```python
from build123d import *

# Parameters (mm, degrees)
BOSS_EXTRUDE2_DEPTH = 6.35
SKETCH6_W           = 2.54
SKETCH6_H           = 7.62
SKETCH6_W_2         = 1.905
CUT_EXTRUDE3_DEPTH  = 6.35
SKETCH7_R           = 10.795
SKETCH7_R_2         = 1.5
CUT_EXTRUDE4_DEPTH  = 6.35
SKETCH10_R          = 7.62
CUT_EXTRUDE6_DEPTH  = 6.35
SKETCH11_W          = 3.81
SKETCH11_H          = 7.62
CUT_EXTRUDE7_DEPTH  = 1.27
SKETCH8_R           = 2
SKETCH8_R_2         = 1.989430384
CUT_EXTRUDE8_DEPTH  = 6.35
SKETCH12_R          = 2
CUT_EXTRUDE9_DEPTH  = 6.35


with BuildPart() as part:
    # Sketch3 → Boss-Extrude2 (new body)
    with BuildSketch(Plane(origin=(0, 0, 0), x_dir=(1, 0, 0), z_dir=(0, 1, 0))):
        with BuildLine():
            Line((-27.819999986, -50.8), (-16.461471842, -50.8))
            Line((-16.461471842, -50.8), (4.000849576, -50.8))
            Line((4.000849576, -50.8), (23.297417358, -50.8))
            Line((23.297417358, -50.8), (27.819999986, -50.8))
            ThreePointArc((27.819999986, -50.8), (29.61605121, -50.056051224), (30.359999986, -48.26))
            Line((30.359999986, -48.26), (30.359999986, -11.643560444))
            ThreePointArc((30.359999986, -11.643560444), (30.670062071, -10.427428504), (31.524548724, -9.508207119))
            ThreePointArc((31.524548724, -9.508207119), (35.329369206, -5.415138673), (36.709999986, 0))
            Line((36.709999986, 0), (36.709999986, 16.964999979))
            ThreePointArc((36.709999986, 16.964999979), (31.054999993, 22.619999972), (25.4, 16.964999979))
            Line((25.4, 16.964999979), (25.4, 11.309999986))
            ThreePointArc((25.4, 11.309999986), (19.514906714, 9.658249153), (15.348771474, 5.185451262))
            ThreePointArc((15.348771474, 5.185451262), (14.413140747, 4.180950232), (13.091466391, 3.81))
            Line((13.091466391, 3.81), (-13.091466391, 3.81))
            ThreePointArc((-13.091466391, 3.81), (-14.413140747, 4.180950232), (-15.348771474, 5.185451262))
            ThreePointArc((-15.348771474, 5.185451262), (-19.514906714, 9.658249153), (-25.4, 11.309999986))
            Line((-25.4, 11.309999986), (-25.4, 16.964999979))
            ThreePointArc((-25.4, 16.964999979), (-31.054999993, 22.619999972), (-36.709999986, 16.964999979))
            Line((-36.709999986, 16.964999979), (-36.709999986, 0))
            ThreePointArc((-36.709999986, 0), (-35.329369206, -5.415138673), (-31.524548724, -9.508207119))
            ThreePointArc((-31.524548724, -9.508207119), (-30.670062071, -10.427428504), (-30.359999986, -11.643560444))
            Line((-30.359999986, -11.643560444), (-30.359999986, -48.26))
            ThreePointArc((-30.359999986, -48.26), (-29.61605121, -50.056051224), (-27.819999986, -50.8))
        make_face()
    extrude(amount=BOSS_EXTRUDE2_DEPTH)

    # Sketch6 → Cut-Extrude3 (cut)
    with BuildSketch(Plane(origin=(0, 6.35, 0), x_dir=(1, 0, 0), z_dir=(0, 1, 0))):
        with Locations((-5.08, -3.81)):
            Rectangle(SKETCH6_W, SKETCH6_H)
        with Locations((4.7625, -3.81)):
            Rectangle(SKETCH6_W_2, SKETCH6_H)
        with Locations((10.4775, -3.81)):
            Rectangle(SKETCH6_W_2, SKETCH6_H)
    extrude(amount=-CUT_EXTRUDE3_DEPTH, mode=Mode.SUBTRACT)

    # Sketch7 → Cut-Extrude4 (cut)
    with BuildSketch(Plane(origin=(0, 6.35, 0), x_dir=(1, 0, 0), z_dir=(0, 1, 0))):
        with Locations((-12.7, -36.83)):
            Circle(SKETCH7_R)
        with Locations((12.7, -36.83)):
            Circle(SKETCH7_R_2)
    extrude(amount=-CUT_EXTRUDE4_DEPTH, mode=Mode.SUBTRACT)

    # Sketch10 → Cut-Extrude6 (cut)
    with BuildSketch(Plane(origin=(0, 6.35, 0), x_dir=(1, 0, 0), z_dir=(0, 1, 0))):
        with Locations((-25.4, 0)):
            Circle(SKETCH10_R)
        with Locations((25.4, 0)):
            Circle(SKETCH10_R)
    extrude(amount=-CUT_EXTRUDE6_DEPTH, mode=Mode.SUBTRACT)

    # Sketch11 → Cut-Extrude7 (cut)
    with BuildSketch(Plane(origin=(0, 6.35, 0), x_dir=(1, 0, 0), z_dir=(0, 1, 0))):
        with Locations((7.62, -3.81)):
            Rectangle(SKETCH11_W, SKETCH11_H)
    extrude(amount=-CUT_EXTRUDE7_DEPTH, mode=Mode.SUBTRACT)

    # Sketch8 → Cut-Extrude8 (cut)
    with BuildSketch(Plane(origin=(0, 6.35, 0), x_dir=(1, 0, 0), z_dir=(0, 1, 0))):
        with Locations((-31.75, 15.24)):
            Circle(SKETCH8_R)
        with Locations((-25.4, -15.24)):
            Circle(SKETCH8_R)
        with Locations((25.4, -15.24)):
            Circle(SKETCH8_R_2)
        with Locations((31.75, 15.24)):
            Circle(SKETCH8_R)
    extrude(amount=-CUT_EXTRUDE8_DEPTH, mode=Mode.SUBTRACT)

    # Sketch12 → Cut-Extrude9 (cut)
    with BuildSketch(Plane(origin=(0, 6.35, 0), x_dir=(1, 0, 0), z_dir=(0, 1, 0))):
        with Locations((15.301414721, -14.889872981)):
            Circle(SKETCH12_R)
        with Locations((20.301414721, -23.550127019)):
            Circle(SKETCH12_R)
        with Locations((-22.133830064, -48.050127019)):
            Circle(SKETCH12_R)
        with Locations((-27.133830064, -39.389872981)):
            Circle(SKETCH12_R)
    extrude(amount=-CUT_EXTRUDE9_DEPTH, mode=Mode.SUBTRACT)


solid = part.part
```
CAD build for the part. Positions are in the model's coordinates, mm. A direction names the side the tool comes from. Coordinates: 2 decimals unless noted, no trailing zeros. Write each loop counter-clockwise with the first axis right and the second up, starting at its lowest first coordinate (ties: lowest second). Pieces come first, ordered by that corner, then holes.
(1) Cut at D-D, the plane x = 24.5. List the corners of the cut face in (y, z).
(2) 3-axis set-ups, long thin cutter, end or side, ignore diameter. For faces 1 (the face through (-1, 6.35, 14)), 2 (the face through (7.6, 5.3, 7.62)), 3 (the face through (25.4, 3, -14)), 4 (the face through (5.715, 3, 4)), 5 (the face through (30.36, 3, 30)): which of +Z, -Z, +X, -X, +Y, -Y reach the whole face in a straight line?
(3) Flat gauge pins, fed straight in: pin 1 (2 mm diameter, centred on y = 2.5, z = 7, fed in from -X); pin 2 (3 mm diameter, centred on y = 2, z = 4, fed in from -X); pin 3 (1 mm diameter, centred on x = -1.5, y = 5.5, fed in from -Z). Where does each tip first touch, or does it go through?
(4) Cut at C-C, the plane x = -22.5. List the corners of the cut face in (y, z), and give its area (3 significant figures).
(5) Cut at B-B, the plane z = 5. List the corners of the cut face in (x, y) (3 decimals).
(6) Cut at A-A, the plane z = -15.24. List the corners of the cut face in (x, y).
(7) Two-plate mould, pull along X, no slides. Class faces 6 (the face through (19.589, 3.131, -9.703)), 7 (the face through (0, 3, 50.8)), 8 (the face through (-35.367, 3.131, 5.346)), 9 (the face through (35.291, 3.131, 5.484)): +X half, -X half, draft (parallel to the pull), parting line (faces both ways), or undercut.
(8) Drill centre lines: probe 1 along X at (y, z) = (3.25, -15.24); probe 2 along X at (y, z) = (4.25, 36.83) (3 decimals); probe 3 along Z at (x, y) = (10, 5.25). Where is each one in solid material? Low to high.
Geometry says:
1. outline: (0, -11.27) - (6.35, -11.27) - (6.35, -7.57) - (0, -7.57) - close; (0, 7.57) - (6.35, 7.57) - (6.35, 13.47) - (0, 13.47) - close; (0, 17.01) - (6.35, 17.01) - (6.35, 50.8) - (0, 50.8) - close
2. face 1: +Z, -Z, +X, -X, +Y
2. face 2: +Y
2. face 3: -Z, +Y, -Y
2. face 4: +Y, -Y
2. face 5: +Z, +X, +Y, -Y
3. pin 1: stops at x = -34.99
3. pin 2: stops at x = -36.43
3. pin 3: stops at z = -3.81
4. outline: (0, -10.93) - (6.35, -10.93) - (6.35, -7.05) - (0, -7.05) - close; (0, 7.05) - (6.35, 7.05) - (6.35, 32.3) - (0, 32.3) - close; (0, 41.36) - (6.35, 41.36) - (6.35, 46.08) - (0, 46.08) - close; (0, 50.02) - (6.35, 50.02) - (6.35, 50.8) - (0, 50.8) - close
4. area: 220 mm2
5. outline: (-35.545, 0) - (-31.15, 0) - (-31.15, 6.35) - (-35.545, 6.35) - close; (-19.65, 0) - (-6.35, 0) - (-6.35, 6.35) - (-19.65, 6.35) - close; (-3.81, 0) - (3.81, 0) - (3.81, 6.35) - (-3.81, 6.35) - close; (5.715, 0) - (9.525, 0) - (9.525, 5.08) - (5.715, 5.08) - close; (11.43, 0) - (19.65, 0) - (19.65, 6.35) - (11.43, 6.35) - close; (31.15, 0) - (35.545, 0) - (35.545, 6.35) - (31.15, 6.35) - close
6. outline: (-36.71, 0) - (-33.75, 0) - (-33.75, 6.35) - (-36.71, 6.35) - close; (-29.75, 0) - (-25.4, 0) - (-25.4, 6.35) - (-29.75, 6.35) - close; (25.4, 0) - (29.75, 0) - (29.75, 6.35) - (25.4, 6.35) - close; (33.75, 0) - (36.71, 0) - (36.71, 6.35) - (33.75, 6.35) - close
7. face 6: undercut
7. face 7: draft
7. face 8: -X half
7. face 9: +X half
8. probe 1: x = -36.71 to -33.75, -29.75 to -25.4, 25.4 to 29.75, 33.75 to 36.71
8. probe 2: x = -30.36 to -23.495, -1.905 to 11.2, 14.2 to 30.36
8. probe 3: z = -3.81 to 0, 7.62 to 50.8
